```python
from build123d import *

# Parameters (mm, degrees)
F1_DEPTH = 50
F2_R     = 2
F3_DEPTH = 25


with BuildPart() as f1:
    # F0 (on Top) → F1 (new body)
    with BuildSketch(Plane.XY):
        with BuildLine():
            ThreePointArc((-10.218003, 18.066239), (-10.082748, 18.408666), (-9.75, 18.566239))
            Line((-9.75, 18.566239), (9.75, 18.566239))
            Line((9.75, 18.566239), (9.749928, 18.565147))
            ThreePointArc((9.749928, 18.565147), (10.093038, 18.395673), (10.215817, 18.03322))
            Line((10.215817, 18.03322), (9.937061, 13.821265))
            Line((9.937061, 13.821265), (9.419089, 13.566239))
            Line((9.419089, 13.566239), (8, -7.875915))
            Line((8, -7.875915), (7, -9.70099))
            Line((7, -9.70099), (8.880575, -13.133215))
            Line((8.880575, -13.133215), (10.666446, -13.015022))
            Line((10.666446, -13.015022), (12.814004, 19.434163))
            ThreePointArc((12.814004, 19.434163), (12.278533, 20.932959), (10.81837, 21.566239))
            Line((10.81837, 21.566239), (-10.81837, 21.566239))
            ThreePointArc((-10.81837, 21.566239), (-12.278533, 20.932959), (-12.814004, 19.434163))
            Line((-12.814004, 19.434163), (-10.658623, -13.133215))
            Line((-10.658623, -13.133215), (-8.866173, -13.133215))
            Line((-8.866173, -13.133215), (-7, -9.625915))
            Line((-7, -9.625915), (-8, -7.875915))
            Line((-8, -7.875915), (-9.419089, 13.566239))
            Line((-9.419089, 13.566239), (-9.937061, 13.821265))
            Line((-9.937061, 13.821265), (-10.218003, 18.066239))
        make_face()
    extrude(amount=F1_DEPTH)

    # F2 (on Right) → F3 (cut)
    with BuildSketch(Plane.YZ):
        with Locations((2.566239, 12.5)):
            Circle(F2_R)
        with Locations((2.566239, 37.5)):
            Circle(F2_R)
    extrude(amount=-F3_DEPTH, mode=Mode.SUBTRACT)


solid = f1.part
```
The listing builds one solid part. Answer for the finished solid, in the listing's coordinates (mm). A direction names the side the tool comes from. Give positions to 0.01 mm unless a question says otherwise; leave off trailing zeros. Order: outer loops, then holes, each group sorted by start corner. A loop starts at its lowest first (then second) coordinate and runs counter-clockwise, first axis right, second up. Notation, with made-up numbers: (21, 60) - (62, 60) arc R26 cw to (62, 96) - close; hole circle Ø10 at (-4, 35.25). An arc over 180 degrees is marked (long way). Answer in a Markdown table with one row per item. Add a question column.
Q1. The part is cut by section A-A (y = -2). Determine the outline of the cut face in (x, z).
Q2. Find the intervals of material crossed by line 1 along Y through (x, z) = (2.25, 22); line 2 along Y through (x, z) = (10.5, 31); line 3 along X through (y, z) = (17.5, 8), in increasing order. Write a range as [from, to].
Q3. Given P1, Ø3, axis at y = 2.57, z = 12.5, coming from the +X side; P2, Ø4.5, axis at y = 2.57, z = 37.5, coming from the -X side; P3, Ø2, axis at y = -0.5, z = 14, coming from the +X side, each flat-ended and moving along its own axis, determine where each tip first touches the part or whether it passes through.
Q4. Which of the six approach directions +Z, -Z, +X, -X, +Y, -Y give full straight-line access (tool end or side, diameter ignored) to faces 4 (the cylindrical face through (-10.17, 0.57, 12.59)), 5 (the flat face through (7.927, -11.393, 24.65)), 6 (the flat face through (8.72, 3, 24.65))?
Q5. The part is cut by section D-D (y = 17). Determine the outline of the cut face in (x, z).
Q6. For a pull along X with two mould halves and no side action, classify faces 1 (the cylindrical face through (-10.17, 0.57, 37.59)), 2 (the flat face through (0, 18.566, 25)), 3 (the flat face through (9.761, -13.075, 24.65)) as released by +X, released by -X, zero draft, split by the parting line, or undercut.
Determined:
| question | item | result |
|---|---|---|
| 1 | outline | (-11.4, 0) - (-8.39, 0) - (-8.39, 50) - (-11.4, 50) - close; (8.39, 0) - (11.4, 0) - (11.4, 50) - (8.39, 50) - close |
| 2 | line 1 | y = [18.57, 21.57] |
| 2 | line 2 | y = [-13.03, 21.57] |
| 2 | line 3 | x = [-12.69, -10.18], [10.18, 12.69] |
| 3 | P1 | stops at x = 11.8 |
| 3 | P2 | stops at x = -11.85 |
| 3 | P3 | stops at x = 11.56 |
| 4 | face 4 | -X |
| 4 | face 5 | +Z, -Z, -Y |
| 4 | face 6 | +Z, -Z |
| 5 | outline | (-12.65, 0) - (-10.15, 0) - (-10.15, 50) - (-12.65, 50) - close; (10.15, 0) - (12.65, 0) - (12.65, 50) - (10.15, 50) - close |
| 6 | face 1 | zero draft |
| 6 | face 2 | undercut |
| 6 | face 3 | released by +X |
